```python
from build123d import *

# Parameters (mm, degrees)
FILLET1_R = 10
FILLET3_R = 10


with BuildPart() as part:
    # Sketch1 → Revolve1 (revolve)
    with BuildSketch(Plane(origin=(0, 0, 0), x_dir=(0, 0, -1), z_dir=(1, 0, 0))):
        with BuildLine():
            Line((-18.394691605, 55.313614898), (-15.803889971, -58.42257686))
            Line((-15.803889971, -58.42257686), (-40.675585663, -58.42257686))
            Line((-40.675585663, -58.42257686), (-40.675585663, -4.274822697))
            ThreePointArc((-40.675585663, -4.274822697), (-31.876602198, -0.630164411), (-28.231943912, 8.168819054))
            Line((-28.231943912, 8.168819054), (-28.231943912, 55.313614898))
            Line((-28.231943912, 55.313614898), (-18.394691605, 55.313614898))
        make_face()
    revolve(axis=Axis((0, 55.313614898, 18.394691605), (0, -0.9997406585155251, -0.02277313572928287)))

    # Fillet1
    fillet1_edges = [part.edges().sort_by_distance(p)[0] for p in [
        (0, -57.290057641, -9.042008017),
    ]]
    fillet(fillet1_edges, radius=FILLET1_R)

    # Fillet3
    fillet3_edges = [part.edges().sort_by_distance(p)[0] for p in [
        (0, -3.198467231, -6.576419302),
    ]]
    fillet(fillet3_edges, radius=FILLET3_R)


solid = part.part
```
The model under review builds one solid part; all positions refer to its coordinate system, in mm. A direction names the side the tool comes from. Give positions to 0.01 mm unless a question says otherwise; leave off trailing zeros.
(1) The part is to be moulded in two halves that separate along X. For faces 1 (the conical face through (6.31, 32.49, 9.65)), 2 (the conical face through (0.291, 55.333, 18.016)), say which applies: released by +X, released by -X, zero draft, split by the parting line, or undercut.
(2) For P1, Ø12, axis at x = -9, y = -15.5, coming from the +Z side; P2, Ø3, axis at y = -29, z = 5, coming from the +X side; P3, Ø8, axis at y = -20, z = 7.5, coming from the +X side; P4, Ø2, axis at x = 13, y = 44.5, coming from the -Z side, all flat-tipped, find the tip position at first contact; note any pin that passes through.
(3) Tool access review of faces 3 (the conical face through (0.36, -58.42, 16.66)), 4 (the conical face through (9.27, -29.88, 38.83)): name each direction out of +Z, -Z, +X, -X, +Y, -Y from which nothing blocks a thin tool from reaching the whole face with its end or side.
(4) To check wall thickness, follow L1, parallel to X at y = -30, z = 12; L2, parallel to Y at x = -17.5, z = 15; L3, parallel to X at y = -12, z = 32. State the ranges of each line that lie inside material, in increasing order.
Returned:
1. face 1: split by the parting line
1. face 2: undercut
2. P1: stops at z = 40.49
2. P2: stops at x = 22.07
2. P3: stops at x = 23.45
2. P4: passes through
3. face 3: -Z, -Y
3. face 4: +Y
4. L1: x = -23.82 to 23.82
4. L2: y = -57.64 to -2.3
4. L3: x = -18.38 to 18.38
